Autodesk Inventor part; units mm, degrees
ref_plane "YZ Plane" through (0, 0, 0) normal (1, 0, 0) x (0, 1, 0)
ref_plane "XZ Plane" through (0, 0, 0) normal (0, 1, 0) x (-1, 0, 0)
ref_plane "XY Plane" through (0, 0, 0) normal (0, 0, 1) x (1, 0, 0)
sketch "Sketch2" plane through (0, 0, 0) normal (0, 0, 1) x (1, 0, 0)
  circle A0 centre (0, 0) radius 75
  dimension "d0" = 150
extrude "Extrusion1" add sketch "Sketch2" along normal blind 10
fillet "Fillet1" radius 2 1 edges at (-75, 0, 10)
fillet "Fillet2" radius 2 1 edges at (-75, 0, 0)
sketch "Sketch24" plane through (0, 0, 0) normal (1, 0, 0) x (0, 1, 0)
  line L0 (10, 0) -> (-10, 0)
  point P0 (0, 0)
sketch "Sketch25" plane through (0, 0, 0) normal (0, 0, 1) x (1, 0, 0)
  circle A0 centre (0, 0) radius 73
  circle A1 centre (23.8125, -61.9125) radius 2.5
  circle A2 centre (51.5785, -41.7115) radius 2.5
  circle A3 centre (65.524, -10.334) radius 2.5
  circle A4 centre (61.9125, 23.8125) radius 2.5
  circle A5 centre (41.7115, 51.5785) radius 2.5
  circle A6 centre (10.334, 65.524) radius 2.5
  circle A7 centre (-23.8125, 61.9125) radius 2.5
  circle A8 centre (-51.5785, 41.7115) radius 2.5
  circle A9 centre (-65.524, 10.334) radius 2.5
  circle A10 centre (-61.9125, -23.8125) radius 2.5
  circle A11 centre (-41.7115, -51.5785) radius 2.5
  circle A12 centre (-10.334, -65.524) radius 2.5
  circle A13 centre (0, 0) radius 10
  circle A14 centre (0, 0) radius 10
  dimension "d104" = 5
  dimension "d107" = 360
sketch "Sketch26" plane through (0, 0, 0) normal (0, 0, -1) x (-1, 0, 0)
  point P0 (0, 0)
extrude "Extrusion6" add sketch "Sketch25" against normal blind 50 contours A2 | A3 | A4 | A5 | A6 | A7 | A8 | A9 | A10 | A11 | A12
sketch "Sketch29" plane through (0, 0, 0) normal (0, 0, 1) x (1, 0, 0)
  circle A0 centre (23.8125, -61.9125) radius 2.5
  point P0 (0, 0)
  dimension "d111" = 5
extrude "Extrusion7" add sketch "Sketch29" against normal blind 50
sketch "Sketch30" plane through (0, 0, 0) normal (0, 0, 1) x (1, 0, 0)
  point P0 (0, 0)
sketch "Sketch31" plane through (0, 0, 0) normal (0, 0, 1) x (1, 0, 0)
  point P0 (0, 0)
sketch "Sketch32" plane through (0, 0, 10) normal (0, 0, 1) x (1, 0, 0)
  circle A0 centre (0, 0) radius 4
  dimension "d114" = 8
extrude "Extrusion8" cut sketch "Sketch32" against normal through all both and the other way through all
sketch "Sketch33" plane through (0, 0, 10) normal (0, 0, 1) x (1, 0, 0)
  circle A0 centre (0, 0) radius 4
  circle A1 centre (0, 0) radius 31.511
extrude "Extrusion9" add sketch "Sketch33" along normal blind 10
fillet "Fillet3" radius 2 1 edges at (-31.511, 0, 20)
sketch "Sketch34" plane through (0, 0, 20) normal (0, 0, 1) x (1, 0, 0)
  circle A0 centre (0, 0) radius 4
  circle A1 centre (0, 0) radius 4.5
  dimension "d120" = 9
extrude "Extrusion10" add sketch "Sketch34" along normal blind 80 contours A0 | A1
sketch "Sketch35" plane through (0, 0, 100) normal (0, 0, 1) x (1, 0, 0)
  circle A0 centre (0, 0) radius 4
  circle A1 centre (0, 0) radius 4
  dimension "d123" = 8
extrude "Extrusion11" cut sketch "Sketch35" against normal blind 10
properties part number "updated_base"
Source: CAD feature listing. Evaluate the final solid. Frame: model axes, mm. A direction names the side the tool comes from. Give positions to 0.01 mm unless a question says otherwise; leave off trailing zeros. Order: outer loops, then holes, each group sorted by start corner. A loop starts at its lowest first (then second) coordinate and runs counter-clockwise, first axis right, second up. Notation, with made-up numbers: (8, 12) -> (55, 12) arc R17 ccw to (55, 19) -> close; hole circle Ø3 at (5, 51). An arc over 180 degrees is marked (long way). Use a Markdown table: item, result.
Q1. Section C-C (z = 56). Return the cut outline in (x, y).
A:
| item | result |
|---|---|
| outline | circle Ø9 at (0, 0) |
Q2. Pull-direction query (Y, two-part tool) for faces 4 (the face through (-40.558, -53.796, -24.65)), 5 (the face through (31, -15, 10)), 6 (the face through (-0.867, 3.905, 9.86)); classes: +Y half, -Y half, draft (parallel to the pull), parting line (faces both ways), or undercut.
A:
| item | result |
|---|---|
| face 4 | parting line |
| face 5 | draft |
| face 6 | undercut |
Q3. Section A-A (x = 0). Return the cut outline in (y, z), and give its area (3 significant figures).
A:
| item | result |
|---|---|
| outline | (-75, 2) arc R2 ccw to (-73, 0) -> (-4, 0) -> (-4, 20) -> (4, 20) -> (4, 0) -> (73, 0) arc R2 ccw to (75, 2) -> (75, 8) arc R2 ccw to (73, 10) -> (31.51, 10) -> (31.51, 18) arc R2 ccw to (29.51, 20) -> (4.5, 20) -> (4.5, 100) -> (4, 100) -> (4, 90) -> (-4, 90) -> (-4, 100) -> (-4.5, 100) -> (-4.5, 20) -> (-29.51, 20) arc R2 ccw to (-31.51, 18) -> (-31.51, 10) -> (-73, 10) arc R2 ccw to (-75, 8) -> close |
| area | 2,610 mm^2 |
Q4. Access query for faces 1 (the face through (-23.22, -21.3, 13.94)), 2 (the face through (64.3, 24.56, -24.65)), 3 (the face through (-62, -24, -50)). Directions: +Z, -Z, +X, -X, +Y, -Y. A direction counts if a zero-diameter tool reaches every point of the face in a straight line with its end or side. Return the directions, or none.
A:
| item | result |
|---|---|
| face 1 | +Z |
| face 2 | -Z |
| face 3 | -Z, +X, -X, +Y, -Y |
Q5. First-contact query: P1, Ø9, axis at x = 0, y = 1, coming from the -Z side; P2, Ø4, axis at x = -1, y = 0.5, coming from the +Z side; P3, Ø4, axis at x = -9.5, y = 22, coming from the +Z side. Flat tips, straight axial feed; report the tip coordinate or a pass-through.
A:
| item | result |
|---|---|
| P1 | z = 0 |
| P2 | z = 90 |
| P3 | z = 20 |
Q6. Material intervals for line 1 (Y direction, x = 0, z = 97.5); line 2 (Z direction, x = 47.5, y = -7); line 3 (X direction, y = 10, z = -34.5), sorted ascending. Write a range as [from, to].
A:
| item | result |
|---|---|
| line 1 | [-4.5, -4], [4, 4.5] |
| line 2 | [0, 10] |
| line 3 | [-68, -63.05] |
